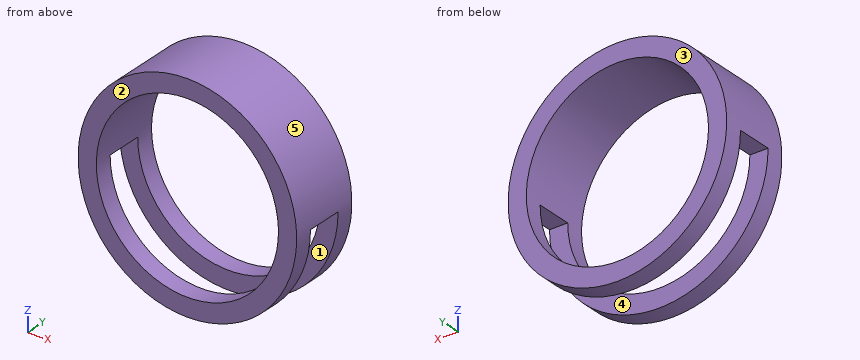
from build123d import *

# Parameters (mm, degrees)
SKETCH1_R           = 30
SKETCH1_R_2         = 25
BOSS_EXTRUDE1_DEPTH = 10
CUT_EXTRUDE1_DEPTH  = 5


with BuildPart() as part:
    # Sketch1 → Boss-Extrude1 (new, symmetric)
    with BuildSketch(Plane(origin=(0, 0, 0), x_dir=(1, 0, 0), z_dir=(0, 1, 0))):
        with Locations(Location((0, 0, 0), (0, 0, 270))):
            Circle(SKETCH1_R)
        with Locations(Location((0, 0, 0), (0, 0, 270))):
            Circle(SKETCH1_R_2, mode=Mode.SUBTRACT)
    extrude(amount=BOSS_EXTRUDE1_DEPTH, both=True)

    # Sketch3 → Cut-Extrude1 (cut, symmetric)
    with BuildSketch(Plane(origin=(0, 0, 0), x_dir=(1, 0, 0), z_dir=(0, 1, 0))):
        with BuildLine():
            ThreePointArc((-25, 0), (0, 25), (25, 0))
            Line((25, 0), (30, 0))
            ThreePointArc((30, 0), (0, 30), (-30, 0))
            Line((-30, 0), (-25, 0))
        make_face()
    extrude(amount=CUT_EXTRUDE1_DEPTH, both=True, mode=Mode.SUBTRACT)


solid = part.part
Can you work these out from the model? Positions are in its coordinate system, mm. Face numbers are marked on the shaded views. A direction names the side the tool comes from. Coordinates: 2 decimals unless noted, no trailing zeros. Write each loop counter-clockwise with the first axis right and the second up, starting at its lowest first coordinate (ties: lowest second). Pieces come first, ordered by that corner, then holes. Notation, with made-up numbers: (32, 89.25) -> (64, 89.25) arc R21 cw to (64, 114.25) -> close; hole circle Ø11 at (66.5, 10.5). An arc over 180 degrees is marked (long way). Write each question's results on one line, items separated by ' | '. Start each with the question number.
Q1. Imagine slicing it at C-C (x = 0). Write out the boundary of the cut face in (y, z), then the cut area to 3 significant figures.
Q2. Imagine slicing it at B-B (y = -6). Write out the boundary of the cut face in (x, z).
Q3. We'd pull the mould along Y, two halves only. Please class the marked faces 1, 2 and 3: +Y half, -Y half, draft (parallel to the pull), parting line (faces both ways), or undercut.
Q4. Imagine slicing it at A-A (x = -24). Write out the boundary of the cut face in (y, z).
Q5. I'm going to push flat-ended pins straight in: pin 1 (1.5 mm diameter, centred on x = -27.5, y = 2.5, fed in from -Z); pin 2 (4 mm diameter, centred on x = 4, y = -0.5, fed in from -Z); pin 3 (1.5 mm diameter, centred on x = -1.5, y = 6, fed in from +Z). Where does each tip first touch, or does it pass through?
Q6. On a 3-axis mill with a long thin cutter (end or side, diameter ignored), from which of +Z, -Z, +X, -X, +Y, -Y can I reach the whole of each face in a straight line? I mean the marked faces 4 and 5. Say none if no direction works.
Q7. If I drill on probe 1 along Y at (x, z) = (-11, -27); probe 2 along X at (y, z) = (-5.5, 0); probe 3 along X at (y, z) = (-1.75, 4), over which ranges is the centre line in solid material (lowest first)?
Taken from the geometry:
1) outline: (-10, -30) -> (-5, -30) -> (-5, -25) -> (-10, -25) -> close; (-10, 25) -> (10, 25) -> (10, 30) -> (-10, 30) -> close; (5, -30) -> (10, -30) -> (10, -25) -> (5, -25) -> close | area: 150 mm^2
2) outline: circle Ø60 at (0, 0); hole circle Ø50 at (0, 0)
3) face 1: undercut | face 2: -Y half | face 3: +Y half
4) outline: (-10, -18) -> (-5, -18) -> (-5, -7) -> (-10, -7) -> close; (-10, 7) -> (10, 7) -> (10, 18) -> (-10, 18) -> close; (5, -18) -> (10, -18) -> (10, -7) -> (5, -7) -> close
5) pin 1: stops at z = 0 | pin 2: stops at z = 24.27 | pin 3: stops at z = 29.99
6) face 4: -Z, +X, -X | face 5: +Y, -Y
7) probe 1: y = -10 to -5, 5 to 10 | probe 2: x = -30 to -25, 25 to 30 | probe 3: x = -29.73 to -24.68, 24.68 to 29.73
